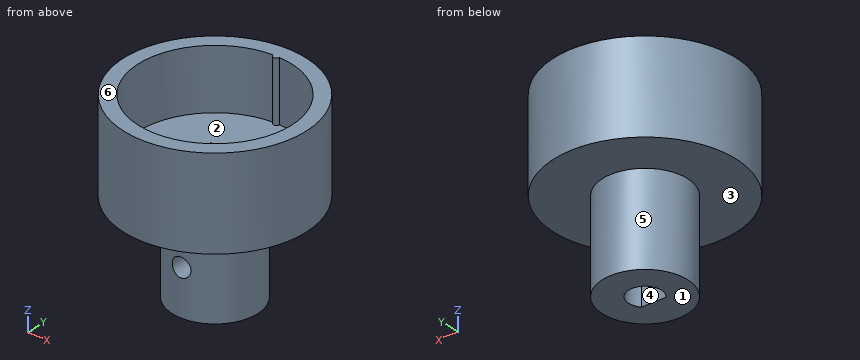
from build123d import *

# Parameters (mm, degrees)
F0_R     = 7
F1_DEPTH = 15
F2_DEPTH = 5
F0_R_2   = 15
F3_DEPTH = 15
F5_D     = 3.1
F5_DEPTH = 13.201
F6_DEPTH = 15
F7_W     = 7
F7_H     = 7
F8_DEPTH = 3


with BuildPart() as f1:
    # F0 (on Top) → F1 (new body)
    with BuildSketch(Plane.XY):
        Circle(F0_R)
        with BuildLine():
            Line((2.0124611797, -1.8), (-2.0124611797, -1.8))
            ThreePointArc((-2.0124611797, -1.8), (0, 2.7), (2.0124611797, -1.8))
        make_face(mode=Mode.SUBTRACT)
    extrude(amount=-F1_DEPTH)

    # F0 (on Top) → F2 (join)
    with BuildSketch(Plane.XY):
        with BuildLine():
            ThreePointArc((-0.4999015713, 12.5900793651), (-8.731014838, -9.0845682286), (12.6, 0))
            ThreePointArc((12.6, 0), (9.0845682286, 8.731014838), (0.4999015713, 12.5900793651))
            ThreePointArc((0.4999015713, 12.5900793651), (0, 12.1), (-0.4999015713, 12.5900793651))
        make_face()
        Circle(F0_R, mode=Mode.SUBTRACT)
        Circle(F0_R)
        with BuildLine():
            Line((2.0124611797, -1.8), (-2.0124611797, -1.8))
            ThreePointArc((-2.0124611797, -1.8), (0, 2.7), (2.0124611797, -1.8))
        make_face(mode=Mode.SUBTRACT)
        with BuildLine():
            ThreePointArc((2.0124611797, -1.8), (0, 2.7), (-2.0124611797, -1.8))
            Line((-2.0124611797, -1.8), (2.0124611797, -1.8))
        make_face()
    extrude(amount=F2_DEPTH)

    # F0 (on Top) → F3 (join)
    with BuildSketch(Plane.XY):
        Circle(F0_R_2)
        with BuildLine():
            ThreePointArc((0.4999015713, 12.5900793651), (9.0845682286, 8.731014838), (12.6, 0))
            ThreePointArc((12.6, 0), (-8.731014838, -9.0845682286), (-0.4999015713, 12.5900793651))
            ThreePointArc((-0.4999015713, 12.5900793651), (0, 12.6), (0.4999015713, 12.5900793651))
        make_face(mode=Mode.SUBTRACT)
    extrude(amount=F3_DEPTH)

    # F5 (through all, one way)
    with BuildSketch(Plane(origin=(0, -1.8, 0), x_dir=(-1, 0, 0), z_dir=(0, 1, 0))):
        with Locations((0, -7.5)):
            Circle(F5_D / 2)
    extrude(amount=-F5_DEPTH, mode=Mode.SUBTRACT)

    # F0 (on Top) → F6 (join)
    with BuildSketch(Plane.XY):
        with BuildLine():
            ThreePointArc((-0.4999015713, 12.5900793651), (0, 12.1), (0.4999015713, 12.5900793651))
            ThreePointArc((0.4999015713, 12.5900793651), (0, 12.6), (-0.4999015713, 12.5900793651))
        make_face()
    extrude(amount=F6_DEPTH)

    # F7 (on face) → F8 (cut)
    with BuildSketch(Plane.XY.offset(5)):
        Rectangle(F7_W, F7_H)
    extrude(amount=-F8_DEPTH, mode=Mode.SUBTRACT)


solid = f1.part
For this review, take the finished solid that the model builds, in its own axes (mm). Face numbers are marked on the shaded views. A direction names the side the tool comes from. Give positions to 0.01 mm unless a question says otherwise; leave off trailing zeros. Loops run counter-clockwise (first coordinate to the right, second up) from the corner with the lowest first, then second, coordinate; pieces in that order, holes last.
Item 1: Insertion check: pin 1 (12 mm diameter, centred on x = 12, y = -0.5, fed in from -Z); pin 2 (0.9 mm diameter, centred on y = -1, z = 3, fed in from -X); pin 3 (1.5 mm diameter, centred on y = 6, z = 3, fed in from +X); pin 4 (3.5 mm diameter, centred on x = -1.5, y = 0.5, fed in from +Z). Each pin has a flat end and moves straight along its axis. Give the tip position at first contact, or say it passes through.
Item 2: Take a section at A-A, the plane x = 0. State the section outline as (y, z) points, and give its area (3 significant figures).
Item 3: Take a section at D-D, the plane y = -9.25. State the section outline as (x, z) points.
Item 4: For line 1 along Z through (x, y) = (0, -5.5); line 2 along Y through (x, z) = (0, 8.75); line 3 along Z through (x, y) = (-7.75, 12.75), list the stretches that pass through material, from the lowest coordinate up.
Item 5: Draft analysis for pull direction Y (two halves, no side actions). For the marked faces 4, 5 and 6, state which applies: +Y half, -Y half, draft (parallel to the pull), parting line (faces both ways), or undercut.
Item 6: Tool access review of the marked faces 1, 2 and 3: name each direction out of +Z, -Z, +X, -X, +Y, -Y from which nothing blocks a thin tool from reaching the whole face with its end or side.
Item 7: Take a section at B-B, the plane z = -9.5. State the section outline as (x, y) points, and give its area (3 significant figures).
Item 8: Take a section at C-C, the plane x = 10. State the section outline as (y, z) points, and give its area (3 significant figures).
Calculated:
1. pin 1: stops at z = -15
1. pin 2: stops at x = -14.99
1. pin 3: stops at x = 14.05
1. pin 4: stops at z = 2
2. outline: (-15, 0) - (-7, 0) - (-7, -5.95) - (-1.8, -5.95) - (-1.8, 0) - (2.7, 0) - (2.7, -15) - (7, -15) - (7, 0) - (15, 0) - (15, 15) - (12.1, 15) - (12.1, 5) - (3.5, 5) - (3.5, 2) - (-3.5, 2) - (-3.5, 5) - (-12.6, 5) - (-12.6, 15) - (-15, 15) - close; (-7, -15) - (-1.8, -15) - (-1.8, -9.05) - (-7, -9.05) - close
2. area: 308 mm2
3. outline: (-11.81, 0) - (11.81, 0) - (11.81, 15) - (8.56, 15) - (8.56, 5) - (-8.56, 5) - (-8.56, 15) - (-11.81, 15) - close
4. line 1: z = -15 to -9.05, -5.95 to 5
4. line 2: y = -15 to -12.6, 12.1 to 15
4. line 3: z = 0 to 15
5. face 4: undercut
5. face 5: parting line
5. face 6: draft
6. face 1: -Z, +X, -X, +Y, -Y
6. face 2: +Z
6. face 3: -Z
7. outline: circle Ø14 at (0, 0); hole (-2.01, -1.8) - (2.01, -1.8) arc R2.7 ccw (long way) to start
7. area: 134 mm2
8. outline: (-11.18, 0) - (11.18, 0) - (11.18, 15) - (7.67, 15) - (7.67, 5) - (-7.67, 5) - (-7.67, 15) - (-11.18, 15) - close
8. area: 182 mm2
